Verification items for the finished model (mm, model axes). Give positions to 0.01 mm unless a question says otherwise; leave off trailing zeros. Order: outer loops, then holes, each group sorted by start corner. A loop starts at its lowest first (then second) coordinate and runs counter-clockwise, first axis right, second up.
from build123d import *

# Parameters (mm, degrees)
SKETCH_1_R      = 76.75
SKETCH_1_R_2    = 1.5
SKETCH_1_R_3    = 2.5
SKETCH_1_W      = 56
SKETCH_1_H      = 115
EXTRUDE_1_DEPTH = 3
FILLET_1_R      = 2


with BuildPart() as part:
    # 草图1 → 凸台-拉伸1 (new body)
    with BuildSketch(Plane(origin=(0, 0, 0), x_dir=(1, 0, 0), z_dir=(0, 1, 0))):
        with Locations(Location((0, 0, 0), (0, 0, 270))):
            Circle(SKETCH_1_R)
        with Locations(Location((0, 72.5, 0), (0, 0, 270))):
            Circle(SKETCH_1_R_2, mode=Mode.SUBTRACT)
        with Locations(Location((51.265241636, 51.265241636, 0), (0, 0, 270))):
            Circle(SKETCH_1_R_2, mode=Mode.SUBTRACT)
        with Locations(Location((72.5, 0, 0), (0, 0, 270))):
            Circle(SKETCH_1_R_2, mode=Mode.SUBTRACT)
        with Locations(Location((51.265241636, -51.265241636, 0), (0, 0, 270))):
            Circle(SKETCH_1_R_2, mode=Mode.SUBTRACT)
        with Locations(Location((0, -72.5, 0), (0, 0, 270))):
            Circle(SKETCH_1_R_2, mode=Mode.SUBTRACT)
        with Locations(Location((-51.265241636, -51.265241636, 0), (0, 0, 270))):
            Circle(SKETCH_1_R_2, mode=Mode.SUBTRACT)
        with Locations(Location((-72.5, 0, 0), (0, 0, 270))):
            Circle(SKETCH_1_R_2, mode=Mode.SUBTRACT)
        with Locations(Location((-51.265241636, 51.265241636, 0), (0, 0, 270))):
            Circle(SKETCH_1_R_2, mode=Mode.SUBTRACT)
        with Locations(Location((-32.5, -20.5, 0), (0, 0, 270))):
            Circle(SKETCH_1_R_2, mode=Mode.SUBTRACT)
        with Locations(Location((-38.5, -20.5, 0), (0, 0, 270))):
            Circle(SKETCH_1_R_2, mode=Mode.SUBTRACT)
        with Locations(Location((-38.5, 20.5, 0), (0, 0, 270))):
            Circle(SKETCH_1_R_2, mode=Mode.SUBTRACT)
        with Locations(Location((-53.5, 25.5, 0), (0, 0, 270))):
            Circle(SKETCH_1_R_3, mode=Mode.SUBTRACT)
        with Locations(Location((-61.5, 25.5, 0), (0, 0, 270))):
            Circle(SKETCH_1_R_3, mode=Mode.SUBTRACT)
        with Locations(Location((-53.5, -25.5, 0), (0, 0, 90))):
            Circle(SKETCH_1_R_3, mode=Mode.SUBTRACT)
        with Locations(Location((-61.5, -25.5, 0), (0, 0, 90))):
            Circle(SKETCH_1_R_3, mode=Mode.SUBTRACT)
        with Locations(Location((-32.5, 20.5, 0), (0, 0, 270))):
            Circle(SKETCH_1_R_2, mode=Mode.SUBTRACT)
        with Locations(Location((35.5, 20.5, 0), (0, 0, 270))):
            Circle(SKETCH_1_R_2, mode=Mode.SUBTRACT)
        with Locations(Location((41.5, 20.5, 0), (0, 0, 270))):
            Circle(SKETCH_1_R_2, mode=Mode.SUBTRACT)
        with Locations(Location((35.5, -20.5, 0), (0, 0, 270))):
            Circle(SKETCH_1_R_2, mode=Mode.SUBTRACT)
        with Locations(Location((41.5, -20.5, 0), (0, 0, 270))):
            Circle(SKETCH_1_R_2, mode=Mode.SUBTRACT)
        Rectangle(SKETCH_1_W, SKETCH_1_H, mode=Mode.SUBTRACT)
    extrude(amount=EXTRUDE_1_DEPTH)

    # 圆角1
    fillet_1_edges = [part.edges().sort_by_distance(p)[0] for p in [
        (28, 1.5, 57.5),
        (28, 1.5, -57.5),
        (-28, 1.5, -57.5),
        (-28, 1.5, 57.5),
    ]]
    fillet(fillet_1_edges, radius=FILLET_1_R)


solid = part.part
(1) Section check A-A, the plane z = 45. Enter the section's corners in (x, y).
Solved:
outline: (-62.17, 0) - (-28, 0) - (-28, 3) - (-62.17, 3) - close; (28, 0) - (62.17, 0) - (62.17, 3) - (28, 3) - close
(2) Scan lines: line 1 (X direction, y = 2.15, z = -20.5); line 2 (X direction, y = 0.85, z = 25.5); line 3 (Z direction, x = -33.5, y = 0.9). Record each from-to range of solid material in increasing order.
Solved:
line 1: x = -73.96 to -40, -37 to -34, -31 to -28, 28 to 34, 37 to 40, 43 to 73.96
line 2: x = -72.39 to -64, -59 to -56, -51 to -28, 28 to 72.39
line 3: z = -69.05 to -21.62, -19.38 to 19.38, 21.62 to 69.05
(3) Section check B-B, the plane y = 1.95. Give the number of separate pieces and of enclosed holes in the cut face, then the cut area to 3 significant figures.
Solved:
separate pieces: 1
enclosed holes: 21
area: 11,900 mm2
(4) Release check for a two-part mould opening along X. For faces 1 (the cylindrical face through (-74.925, 1.479, -16.638)), 2 (the flat face through (-33, 3, -1)), 3 (the cylindrical face through (-59.81, 1.48, -27.34)) record: pulls with the +X half, pulls with the -X half, needs draft (parallel to the pull), parting line crosses it, or undercut.
Solved:
face 1: parting line crosses it
face 2: needs draft
face 3: undercut
(5) Section check C-C, the plane x = 10. Enter the section's corners in (y, z), then the cut area to 3 significant figures.
Solved:
outline: (0, -76.1) - (3, -76.1) - (3, -57.5) - (0, -57.5) - close; (0, 57.5) - (3, 57.5) - (3, 76.1) - (0, 76.1) - close
area: 112 mm2
(6) Go/stop test with flat-tipped pins: pin 1 (0.9 mm diameter, centred on y = 1, z = 11.5, fed in from +X); pin 2 (1 mm diameter, centred on x = 48, y = 2.5, fed in from +Z); pin 3 (1 mm diameter, centred on y = 1, z = -4, fed in from +X). Record where each tip stops, or that it passes through.
Solved:
pin 1: stops at x = 75.95
pin 2: stops at z = 60.29
pin 3: stops at x = 76.67
(7) Section check D-D, the plane x = 46. Enter the section's corners in (y, z).
Solved:
outline: (0, -61.44) - (3, -61.44) - (3, 61.44) - (0, 61.44) - close
